Check sheet for the modelled part. Datum: model origin and axes. Units: mm. Face numbers are marked on the shaded views. A direction names the side the tool comes from. Round coordinates to 2 decimals unless told otherwise and drop trailing zeros. Loops run counter-clockwise (first coordinate to the right, second up) from the corner with the lowest first, then second, coordinate; pieces in that order, holes last. Notation, with made-up numbers: (29.25, 45.5) - (82.25, 45.5) arc R18 cw to (82.25, 75.5) - close; hole circle Ø5 at (-16.5, 23). An arc over 180 degrees is marked (long way). Answer in a Markdown table with one row per item. Add a question column.
(1) Cross-section at A-A on x = 1.5. Count the separate pieces of the cut face and the enclosed holes in it, then the cut area to 3 significant figures.
(2) Thickness scan on line 1 along Y through (x, z) = (43.5, -9.1); line 2 along Y through (x, z) = (7, -3.75); line 3 along Y through (x, z) = (6, -9.25). Record the ranges inside material, lowest first.
(3) Gauge pin test, flat ends, axial feed: pin 1 (5.5 mm diameter, centred on x = 22, z = -3.5, fed in from -Y); pin 2 (6 mm diameter, centred on x = 25, y = -15.5, fed in from -Z); pin 3 (5.5 mm diameter, centred on x = 26, z = -3, fed in from +Y). Record the tip position at first contact, or that the pin passes through.
(4) Cross-section at B-B on z = -9.5. Enter the section's corners in (x, y).
(5) Cross-section at C-C on y = -10. Enter the section's corners in (x, z).
(6) Access from +Z, -Z, +X, -X, +Y, -Y to the whole of each face (thin tool, end or side, straight path). Record for the marked faces 5, 6 and 7.
(7) Cross-section at D-D on x = 36. Enter the section's corners in (y, z).
(8) Mould release check, pull along Y, two halves, no side actions. Record for the marked faces 1, 2, 3 and 4: +Y half, -Y half, draft (parallel to the pull), parting line (faces both ways), or undercut.
Autodesk Inventor part; units mm, degrees
ref_plane "YZ Plane" through (0, 0, 0) normal (1, 0, 0) x (0, 1, 0)
ref_plane "XZ Plane" through (0, 0, 0) normal (0, 1, 0) x (-1, 0, 0)
ref_plane "XY Plane" through (0, 0, 0) normal (0, 0, 1) x (1, 0, 0)
sketch "Sketch1" plane through (0, 0, 0) normal (0, 0, 1) x (1, 0, 0)
  circle A0 centre (36, -10) radius 0.8353
  circle A1 centre (9, -10) radius 0.8353
  circle A2 centre (1.5, -1.5) radius 1
  circle A3 centre (1.5, -18.5) radius 1
  circle A4 centre (43.5, -1.5) radius 1
  circle A5 centre (43.5, -18.5) radius 1
  line L0 (0, -20) -> (45, -20)
  line L1 (45, -20) -> (45, 0)
  line L2 (45, 0) -> (0, 0)
  line L3 (0, 0) -> (0, -20)
  circle A6 centre (36, -10) radius 8.5
  line L4 (46, 1) -> (-1, 1)
  line L5 (-1, 1) -> (-1, -21)
  line L6 (-1, -21) -> (46, -21)
  line L7 (46, -21) -> (46, 1)
  circle A7 centre (9, -10) radius 8.5
  circle A8 centre (36, -10) radius 8
  circle A9 centre (9, -10) radius 8
  dimension "d0" = 17
  dimension "d1" = 47
  dimension "d2" = 22
  dimension "d3" = 1
  dimension "d4" = 1
  dimension "d5" = 17
extrude "Extrusion1" add sketch "Sketch1" along normal blind 3 contours L3 L2 L1 L0 | L7 L6 L5 L4
sketch "Sketch5" plane through (46, -21, 0) normal (1, 0, 0) x (0, 0, -1)
  line L0 (-3, 0) -> (11, 0)
  line L1 (11, -3) -> (-3, -3)
  line L2 (-3, -3) -> (-3, 0)
  line L3 (11, -3) -> (14, -3)
  line L4 (14, -3) -> (14, 22)
  line L5 (14, 22) -> (11, 22)
  line L6 (11, 22) -> (11, 0)
  point P0 (0, 21)
  dimension "d12" = 3
  dimension "d14" = 3
  dimension "d15" = 22
extrude "Extrusion2" add sketch "Sketch5" against normal blind 47
sketch "Sketch6" plane through (46, -24, -14) normal (0, 0, -1) x (-1, 0, 0)
  circle A0 centre (2.5, 22.5) radius 1
  circle A1 centre (44.5, 22.5) radius 1
  circle A2 centre (44.5, 5.5) radius 1
  circle A3 centre (2.5, 5.5) radius 1
  line L0 (0, 25) -> (47, 25)
  line L1 (42, 25) -> (5, 25)
  line L2 (5, 25) -> (5, 5)
  line L3 (5, 5) -> (42, 5)
  line L4 (42, 5) -> (42, 25)
  line L5 (47, 25) -> (47, 0)
  line L6 (0, 25) -> (0, 0)
  line L7 (0, 0) -> (47, 0)
  point P0 (46, 24)
  dimension "d18" = 5
  dimension "d19" = 5
  dimension "d20" = 5
extrude "Extrusion3" cut sketch "Sketch6" against normal up to surface (3 mm away) contours L0 L4 L3 L2
sketch "Sketch8" plane through (46, 1, -11) normal (0, 1, 0) x (1, 0, 0)
  line L0 (0, 3) -> (-47, 3)
  line L1 (-47, 3) -> (-47, -14)
  line L2 (-47, -14) -> (0, -14)
  line L3 (0, -14) -> (0, 3)
  point P0 (-46, -11)
  point P1 (0, -14)
extrude "Extrusion4" add sketch "Sketch8" along normal blind 3
sketch "Sketch9" plane through (46, -24, -14) normal (0, 0, -1) x (-1, 0, 0)
  line L0 (0, 28) -> (47, 28)
  line L1 (0, 0) -> (0, 28)
  line L2 (47, 0) -> (47, 28)
  line L3 (0, 0) -> (47, 0)
  point P0 (46, 24)
extrude "Extrusion5" cut sketch "Sketch9" against normal blind 3
sketch "Sketch10" plane through (46, 4, -11) normal (0, 1, 0) x (1, 0, 0)
  line L0 (-47, 0) -> (0, 0)
  line L1 (0, 0) -> (0, -3)
  line L2 (0, -3) -> (-47, -3)
  line L3 (-47, -3) -> (-47, 0)
  point P0 (-46, -11)
  dimension "d27" = 3
extrude "Extrusion6" add sketch "Sketch10" along normal blind 5
sketch "Sketch11" plane through (-1, -24, 3) normal (0, -1, 0) x (1, 0, 0)
  line L0 (47, -14) -> (0, -14)
  line L1 (0, -14) -> (0, -11)
  line L2 (0, -11) -> (47, -11)
  line L3 (47, -11) -> (47, -14)
  point P0 (1, -3)
  dimension "d30" = 3
extrude "Extrusion7" add sketch "Sketch11" along normal blind 5
sketch "Sketch12" plane through (46, -24, -11) normal (0, 0, -1) x (-1, 0, 0)
  circle A0 centre (2.5, 22.5) radius 1
  circle A1 centre (2.5, 5.5) radius 1
  circle A2 centre (44.5, 22.5) radius 1
  circle A3 centre (44.5, 5.5) radius 1
  circle A4 centre (2.5, 30.5108) radius 1.0033
  line L0 (0, 25) -> (0, 33)
  line L1 (0, 33) -> (47, 33)
  circle A5 centre (44.5, 30.5108) radius 1
  circle A6 centre (44.5, -2.5108) radius 1.0033
  circle A7 centre (2.5, -2.0468) radius 1.0033
  line L2 (47, -5) -> (0, -5)
  point P0 (46, 24)
  dimension "d36" = 2.0066
  dimension "d37" = 2.0066
  dimension "d38" = 2.4892
extrude "Extrusion8" cut sketch "Sketch12" against normal up to next contours A4 | A5 | A6 | A7
properties part number "ProxSensor_Bracket"
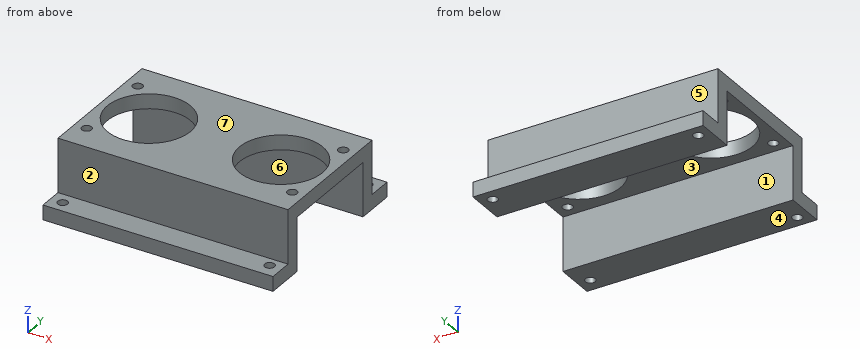
Answers:
| question | item | result |
|---|---|---|
| 1 | separate pieces | 6 |
| 1 | enclosed holes | 0 |
| 1 | area | 132 mm^2 |
| 2 | line 1 | y = -29 to -27.05, -25.04 to -21, 1 to 5.51, 7.51 to 9 |
| 2 | line 2 | y = -24 to -21, 1 to 4 |
| 2 | line 3 | y = -29 to -21, 1 to 9 |
| 3 | pin 1 | stops at y = -24 |
| 3 | pin 2 | stops at z = 0 |
| 3 | pin 3 | stops at y = 4 |
| 4 | outline | (-1, -29) - (46, -29) - (46, -21) - (-1, -21) - close; (-1, 1) - (46, 1) - (46, 9) - (-1, 9) - close; hole circle Ø2.01 at (1.5, -26.51); hole circle Ø2 at (1.5, 6.51); hole circle Ø2.01 at (43.5, -26.05); hole circle Ø2.01 at (43.5, 6.51) |
| 5 | outline | (-1, 0) - (0.5, 0) - (0.5, 3) - (-1, 3) - close; (17.5, 0) - (27.5, 0) - (27.5, 3) - (17.5, 3) - close; (44.5, 0) - (46, 0) - (46, 3) - (44.5, 3) - close |
| 6 | face 5 | +Z, +X, -X, +Y |
| 6 | face 6 | -Z, +X, -X |
| 6 | face 7 | +Z, +X, -X, +Y, -Y |
| 7 | outline | (-29, -11) - (-21, -11) - (-21, 0) - (-18.5, 0) - (-18.5, 3) - (-24, 3) - (-24, -8) - (-29, -8) - close; (-1.5, 0) - (1, 0) - (1, -11) - (9, -11) - (9, -8) - (4, -8) - (4, 3) - (-1.5, 3) - close |
| 8 | face 1 | undercut |
| 8 | face 2 | -Y half |
| 8 | face 3 | undercut |
| 8 | face 4 | draft |
